Design review of the part built by this model. Coordinates are the model's own, in mm. Face numbers are marked on the shaded views. A direction names the side the tool comes from. Coordinates: 2 decimals unless noted, no trailing zeros. Order: outer loops, then holes, each group sorted by start corner. A loop starts at its lowest first (then second) coordinate and runs counter-clockwise, first axis right, second up. Notation, with made-up numbers: M 2,84.25 L 23,84.25 A20 cw 23,101.25 Z; hole C 24.25,-8 d4. An arc over 180 degrees is marked long. Answer as a JSON object with one key per item and string values.
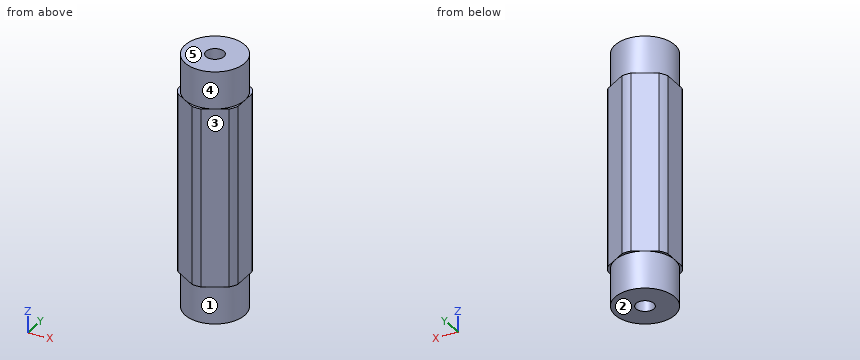
from build123d import *

# Parameters (mm, degrees)
BOSS_EXTRUDE1_DEPTH                  = 26.9748
CUT_EXTRUDE_THIN1_DEPTH              = 29.548108502
CUT_EXTRUDE_THIN1_DEPTH_BACK         = 7.9375
CUT_EXTRUDE_THIN1_START              = 26.9748
SKETCH2_R                            = 8.89
SKETCH2_R_2                          = 6.35
CUT_EXTRUDE_THIN2_START              = -26.9748
SKETCH2_2_R                          = 8.89
SKETCH2_2_R_2                        = 6.35
CUT_EXTRUDE_THIN2_DEPTH              = 7.9375
F_10_24_TAPPED_HOLE1_D               = 3.7973
F_10_24_TAPPED_HOLE1_DEPTH           = 11.938
F_10_24_TAPPED_HOLE1_TIP             = 1.140824014
F_10_24_TAPPED_HOLE1_ON_FACE_2_D     = 3.7973
F_10_24_TAPPED_HOLE1_ON_FACE_2_DEPTH = 11.938
F_10_24_TAPPED_HOLE1_ON_FACE_2_TIP   = 1.140824014


with BuildPart() as part:
    # Sketch1 → Boss-Extrude1 (new, symmetric)
    with BuildSketch(Plane.XY):
        with BuildLine():
            ThreePointArc((0.93173274, 6.79441227), (0, 6.858), (-0.93173274, 6.79441227))
            Line((-0.93173274, 6.79441227), (-5.41826726, 4.204110358))
            ThreePointArc((-5.41826726, 4.204110358), (-5.939202219, 3.429), (-6.35, 2.590301913))
            Line((-6.35, 2.590301913), (-6.35, -2.590301913))
            ThreePointArc((-6.35, -2.590301913), (-5.939202219, -3.429), (-5.41826726, -4.204110358))
            Line((-5.41826726, -4.204110358), (-0.93173274, -6.79441227))
            ThreePointArc((-0.93173274, -6.79441227), (0, -6.858), (0.93173274, -6.79441227))
            Line((0.93173274, -6.79441227), (5.41826726, -4.204110358))
            ThreePointArc((5.41826726, -4.204110358), (5.939202219, -3.429), (6.35, -2.590301913))
            Line((6.35, -2.590301913), (6.35, 2.590301913))
            ThreePointArc((6.35, 2.590301913), (5.939202219, 3.429), (5.41826726, 4.204110358))
            Line((5.41826726, 4.204110358), (0.93173274, 6.79441227))
        make_face()
    extrude(amount=BOSS_EXTRUDE1_DEPTH, both=True)

    # Sketch2 → Cut-Extrude-Thin1 (cut, two sides: drawn at the far end of the back side and taken through both)
    with BuildSketch(Plane.XY.offset(CUT_EXTRUDE_THIN1_START - CUT_EXTRUDE_THIN1_DEPTH_BACK)):
        Circle(SKETCH2_R)
        Circle(SKETCH2_R_2, mode=Mode.SUBTRACT)
    extrude(amount=CUT_EXTRUDE_THIN1_DEPTH + CUT_EXTRUDE_THIN1_DEPTH_BACK, mode=Mode.SUBTRACT)

    # Sketch2<2> → Cut-Extrude-Thin2 (cut)
    with BuildSketch(Plane.XY.offset(CUT_EXTRUDE_THIN2_START)):
        Circle(SKETCH2_2_R)
        Circle(SKETCH2_2_R_2, mode=Mode.SUBTRACT)
    extrude(amount=CUT_EXTRUDE_THIN2_DEPTH, mode=Mode.SUBTRACT)

    # #10-24 Tapped Hole1
    with Locations(Plane.XY.offset(26.9748)):
        with Locations((0, 0)):
            Hole(F_10_24_TAPPED_HOLE1_D / 2, depth=F_10_24_TAPPED_HOLE1_DEPTH)
            with Locations((0, 0, -(F_10_24_TAPPED_HOLE1_DEPTH + F_10_24_TAPPED_HOLE1_TIP / 2))):  # 118° drill point
                Cone(0, F_10_24_TAPPED_HOLE1_D / 2, F_10_24_TAPPED_HOLE1_TIP, mode=Mode.SUBTRACT)

    # #10-24 Tapped Hole1 on face 2
    with Locations(Plane(origin=(0, 0, -26.9748), x_dir=(-1, 0, 0), z_dir=(0, 0, -1))):
        with Locations((0, 0)):
            Hole(F_10_24_TAPPED_HOLE1_ON_FACE_2_D / 2, depth=F_10_24_TAPPED_HOLE1_ON_FACE_2_DEPTH)
            with Locations((0, 0, -(F_10_24_TAPPED_HOLE1_ON_FACE_2_DEPTH + F_10_24_TAPPED_HOLE1_ON_FACE_2_TIP / 2))):  # 118° drill point
                Cone(0, F_10_24_TAPPED_HOLE1_ON_FACE_2_D / 2, F_10_24_TAPPED_HOLE1_ON_FACE_2_TIP, mode=Mode.SUBTRACT)


solid = part.part
1) Add section C-C (x = 4). State the section outline as (y, z) points, and give its area (3 significant figures).
Taken from the geometry:
{"outline": "M -5.02,-19.04 L -4.93,-19.04 L -4.93,-26.97 L 4.93,-26.97 L 4.93,-19.04 L 5.02,-19.04 L 5.02,19.04 L 4.93,19.04 L 4.93,26.97 L -4.93,26.97 L -4.93,19.04 L -5.02,19.04 Z", "area": "539 mm2"}
2) Mouldability with a two-part tool opening along Y and no side actions: class the marked faces 3, 4 and 5 as released by +Y, released by -Y, zero draft, split by the parting line, or undercut.
Taken from the geometry:
{"face 3": "released by -Y", "face 4": "split by the parting line", "face 5": "zero draft"}
3) Insertion check: pin 1 Ø1.5 at (y, z) = (-3.5, -3) entering from -X; pin 2 Ø5 at (x, z) = (3.5, -9.5) entering from -Y (3 decimals); pin 3 Ø3 at (y, z) = (5, 9) entering from -X. Each pin has a flat end and moves straight along its axis. Give the tip position at first contact, or say it passes through.
Taken from the geometry:
{"pin 1": "stops at x = -6.28", "pin 2": "stops at y = -6.755", "pin 3": "stops at x = -5.9"}
4) To check wall thickness, follow L1, parallel to X at y = 0, z = 20.5; L2, parallel to X at y = -0.5, z = 23.5. State the ranges of each line that lie inside material, in increasing order.
Taken from the geometry:
{"L1": "x = -6.35 to -1.9, 1.9 to 6.35", "L2": "x = -6.33 to -1.83, 1.83 to 6.33"}
5) Add section B-B (z = 2). State the section outline as (x, y) points.
Taken from the geometry:
{"outline": "M -6.35,-2.59 A6.86 ccw -5.42,-4.2 L -0.93,-6.79 A6.86 ccw 0.93,-6.79 L 5.42,-4.2 A6.86 ccw 6.35,-2.59 L 6.35,2.59 A6.86 ccw 5.42,4.2 L 0.93,6.79 A6.86 ccw -0.93,6.79 L -5.42,4.2 A6.86 ccw -6.35,2.59 Z"}
6) Tool access review of the marked faces 1 and 2: name each direction out of +Z, -Z, +X, -X, +Y, -Y from which nothing blocks a thin tool from reaching the whole face with its end or side.
Taken from the geometry:
{"face 1": "-Z", "face 2": "-Z, +X, -X, +Y, -Y"}
7) Add section A-A (z = 16). State the section outline as (x, y) points, and give its area (3 significant figures).
Taken from the geometry:
{"outline": "M -6.35,-2.59 A6.86 ccw -5.42,-4.2 L -0.93,-6.79 A6.86 ccw 0.93,-6.79 L 5.42,-4.2 A6.86 ccw 6.35,-2.59 L 6.35,2.59 A6.86 ccw 5.42,4.2 L 0.93,6.79 A6.86 ccw -0.93,6.79 L -5.42,4.2 A6.86 ccw -6.35,2.59 Z; hole C 0,0 d3.8", "area": "126 mm2"}
